```python
from build123d import *

# Parameters (mm, degrees)
SKETCH2_W           = 80
SKETCH2_H           = 60
BOSS_EXTRUDE1_DEPTH = 10
SKETCH3_W           = 40.2
SKETCH3_H           = 19.7
CUT_EXTRUDE1_DEPTH  = 10
FILLET1_R           = 10
SKETCH4_R           = 2.5
SKETCH4_R_2         = 1.6
BOSS_EXTRUDE2_DEPTH = 5
CUT_EXTRUDE2_START  = -21
SKETCH5_R           = 1.6
CUT_EXTRUDE2_DEPTH  = 21
SKETCH7_W           = 55
SKETCH7_H           = 2
CUT_EXTRUDE3_DEPTH  = 2
CUT_EXTRUDE4_DEPTH  = 3


with BuildPart() as part:
    # Sketch2 → Boss-Extrude1 (new body)
    with BuildSketch(Plane(origin=(0, 0, 0), x_dir=(1, 0, 0), z_dir=(0, 1, 0))):
        Rectangle(SKETCH2_W, SKETCH2_H)
    extrude(amount=BOSS_EXTRUDE1_DEPTH)

    # Sketch3 → Cut-Extrude1 (cut)
    with BuildSketch(Plane(origin=(0, 10, 0), x_dir=(1, 0, 0), z_dir=(0, 1, 0))):
        with Locations((-9.9, -2.15)):
            Rectangle(SKETCH3_W, SKETCH3_H)
    extrude(amount=-CUT_EXTRUDE1_DEPTH, mode=Mode.SUBTRACT)

    # Fillet1
    fillet1_edges = [part.edges().sort_by_distance(p)[0] for p in [
        (40, 5, 30),
        (-40, 5, 30),
    ]]
    fillet(fillet1_edges, radius=FILLET1_R)

    # Sketch4 → Boss-Extrude2 (add)
    # profile 1 of 3: a face of its own
    with BuildSketch(Plane(origin=(0, 10, 0), x_dir=(1, 0, 0), z_dir=(0, 1, 0))):
        with Locations(Location((28.2, -2.15, 0), (0, 0, 90))):
            Circle(SKETCH4_R)
        with Locations(Location((28.2, -2.15, 0), (0, 0, 270))):
            Circle(SKETCH4_R_2, mode=Mode.SUBTRACT)
    # profile 2 of 3: a face of its own
    with BuildSketch(Plane(origin=(0, 10, 0), x_dir=(1, 0, 0), z_dir=(0, 1, 0))):
        with Locations(Location((0, -23, 0), (0, 0, 90))):
            Circle(SKETCH4_R)
        with Locations(Location((0, -23, 0), (0, 0, 270))):
            Circle(SKETCH4_R_2, mode=Mode.SUBTRACT)
    # profile 3 of 3: a face of its own
    with BuildSketch(Plane(origin=(0, 10, 0), x_dir=(1, 0, 0), z_dir=(0, 1, 0))):
        with Locations(Location((28.2, -23, 0), (0, 0, 90))):
            Circle(SKETCH4_R)
        with Locations(Location((28.2, -23, 0), (0, 0, 270))):
            Circle(SKETCH4_R_2, mode=Mode.SUBTRACT)
    extrude(amount=BOSS_EXTRUDE2_DEPTH)

    # Sketch5 → Cut-Extrude2 (cut)
    with BuildSketch(Plane(origin=(0, 10, 0), x_dir=(1, 0, 0), z_dir=(0, 1, 0)).offset(CUT_EXTRUDE2_START)):
        with Locations(Location((0, -23, 0), (0, 0, 90))):
            Circle(SKETCH5_R)
        with Locations(Location((28.2, -23, 0), (0, 0, 90))):
            Circle(SKETCH5_R)
        with Locations(Location((28.2, -2.15, 0), (0, 0, 90))):
            Circle(SKETCH5_R)
    extrude(amount=CUT_EXTRUDE2_DEPTH, mode=Mode.SUBTRACT)

    # Sketch7 → Cut-Extrude3 (cut)
    with BuildSketch(Plane.XZ):
        with Locations((-9.9, 2.15)):
            Rectangle(SKETCH7_W, SKETCH7_H)
    extrude(amount=-CUT_EXTRUDE3_DEPTH, mode=Mode.SUBTRACT)

    # Sketch8 → Cut-Extrude4 (cut)
    with BuildSketch(Plane.XZ):
        Polygon((3.464101615, 23), (1.732050808, 26), (-1.732050808, 26), (-3.464101615, 23), (-1.732050808, 20), (1.732050808, 20), align=None)
        Polygon((31.664101615, 23), (29.932050808, 26), (26.467949192, 26), (24.735898385, 23), (26.467949192, 20), (29.932050808, 20), align=None)
        Polygon((31.664101615, 2.15), (29.932050808, 5.15), (26.467949192, 5.15), (24.735898385, 2.15), (26.467949192, -0.85), (29.932050808, -0.85), align=None)
    extrude(amount=-CUT_EXTRUDE4_DEPTH, mode=Mode.SUBTRACT)


solid = part.part
```
CAD build for the part. Positions are in the model's coordinates, mm. A direction names the side the tool comes from. Coordinates: 2 decimals unless noted, no trailing zeros. Write each loop counter-clockwise with the first axis right and the second up, starting at its lowest first coordinate (ties: lowest second). Pieces come first, ordered by that corner, then holes. Notation, with made-up numbers: (77.5, 63.5) -> (93.5, 63.5) arc R24 ccw to (93.5, 82.5) -> close; hole circle Ø8 at (31.5, -20.5). An arc over 180 degrees is marked (long way). Return JSON: item names as keys, results as strings. Group by question number.
Q1. Cut at D-D, the plane x = -24. Give the cut face in (y, z).
Q2. Cut at C-C, the plane y = 5.25. Give the cut face in (x, z).
Q3. Pull direction Z, two halves, no side cores. Call faces 1 (the face through (-40, 5, -5)), 2 (the face through (2.6, 1.5, 24.5)): released by +Z, released by -Z, zero draft, split by the parting line, or undercut.
Q4. Flat gauge pins, fed straight in: pin 1 (1.9 mm diameter, centred on x = 0, z = 23, fed in from +Y) (3 decimals); pin 2 (1.5 mm diameter, centred on x = -2, z = -18, fed in from -Y); pin 3 (1 mm diameter, centred on x = 14.5, z = 2, fed in from -Y); pin 4 (3.5 mm diameter, centred on x = 28.2, z = 23, fed in from -Y). Where does each tip first touch, or does it go through?
Q5. Which spindle directions (+Z, -Z, +X, -X, +Y, -Y) get a long thin tool onto all of the face, cutting with end or side? Do faces 3 (the face through (30.64, 12.46, 2.69)), 4 (the face through (-10, 5, 12)), 5 (the face through (0, 1, 20)). Say none if no direction does.
Q6. Cut at A-A, the plane z = -5. Give the cut face in (x, y), then the cut area to 3 significant figures.
Q7. Cut at B-B, the plane x = 28.2. Give the cut face in (y, z).
Q8. Drill centre lines: line 1 (Z direction, x = 28.2, y = 8.75); line 2 (X direction, y = 11.75, z = 23); line 3 (Z direction, x = -1, y = 7.25). Where is each one in solid material? Low to high.
Returned:
{
 "1": {"outline": "(0, -30) -> (10, -30) -> (10, -7.7) -> (0, -7.7) -> close; (0, 12) -> (10, 12) -> (10, 30) -> (0, 30) -> close"},
 "2": {"outline": "(-40, -30) -> (40, -30) -> (40, 20) arc R10 ccw to (30, 30) -> (-30, 30) arc R10 ccw to (-40, 20) -> close; hole (-30, -7.7) -> (10.2, -7.7) -> (10.2, 12) -> (-30, 12) -> close; hole circle Ø3.2 at (0, 23); hole circle Ø3.2 at (28.2, 2.15); hole circle Ø3.2 at (28.2, 23)"},
 "3": {"face 1": "zero draft", "face 2": "undercut"},
 "4": {"pin 1": "passes through", "pin 2": "stops at y = 0", "pin 3": "stops at y = 2", "pin 4": "stops at y = 3"},
 "5": {"face 3": "+Y", "face 4": "+Y, -Y", "face 5": "-Y"},
 "6": {"outline": "(-40, 0) -> (-30, 0) -> (-30, 10) -> (-40, 10) -> close; (10.2, 0) -> (40, 0) -> (40, 10) -> (10.2, 10) -> close", "area": "398 mm2"},
 "7": {"outline": "(0, -30) -> (10, -30) -> (10, -0.35) -> (15, -0.35) -> (15, 0.55) -> (3, 0.55) -> (3, -0.85) -> (0, -0.85) -> close; (0, 5.15) -> (3, 5.15) -> (3, 3.75) -> (15, 3.75) -> (15, 4.65) -> (10, 4.65) -> (10, 20.5) -> (15, 20.5) -> (15, 21.4) -> (3, 21.4) -> (3, 20) -> (0, 20) -> close; (0, 26) -> (3, 26) -> (3, 24.6) -> (15, 24.6) -> (15, 25.5) -> (10, 25.5) -> (10, 30) -> (0, 30) -> close"},
 "8": {"line 1": "z = -30 to 0.55, 3.75 to 21.4, 24.6 to 30", "line 2": "x = -2.5 to -1.6, 1.6 to 2.5, 25.7 to 26.6, 29.8 to 30.7", "line 3": "z = -30 to -7.7, 12 to 21.75, 24.25 to 30"}
}
